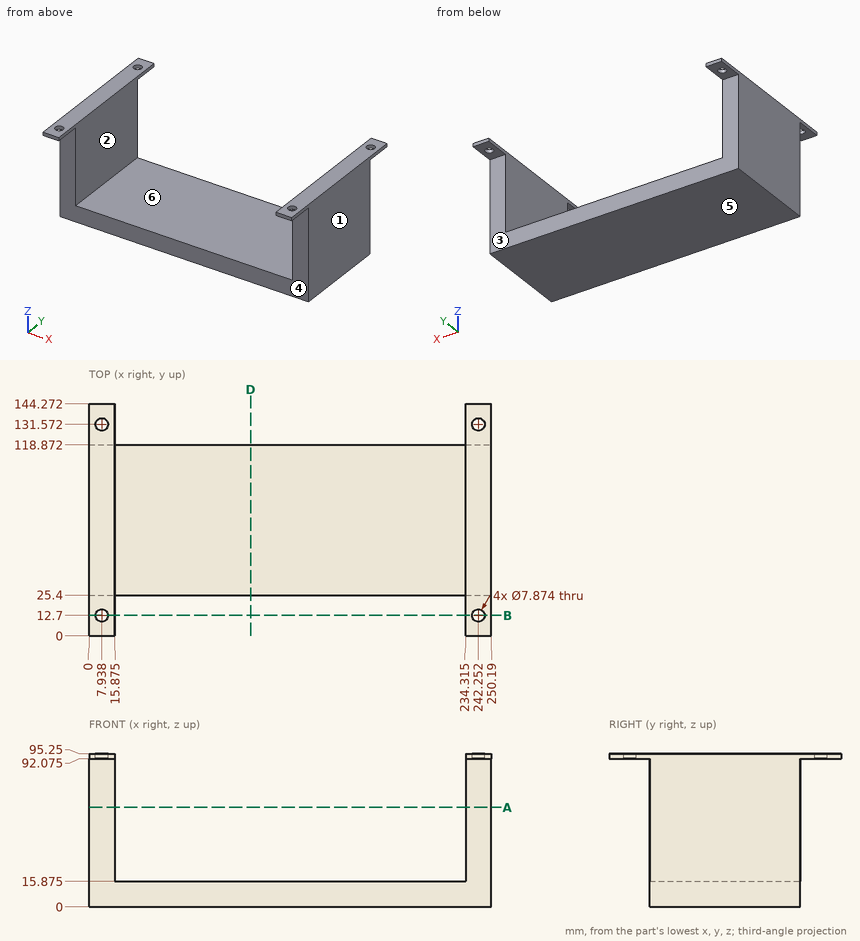
Input: dimensioned drawing with shaded views. Units: mm. Origin: part minimum x, y, z. A direction names the side the tool comes from. Give positions to 0.01 mm unless a question says otherwise; leave off trailing zeros. Loops run counter-clockwise (first coordinate to the right, second up) from the corner with the lowest first, then second, coordinate; pieces in that order, holes last. Notation, with made-up numbers: (-32.5, -17.75) -> (-21.5, -17.75) arc R21 cw to (-21.5, 16.25) -> close; hole circle Ø4 at (-13.5, -15.5). An arc over 180 degrees is marked (long way). Use a Markdown table: item, result.
Q1. Section query B-B, the plane y = 12.7. State how many separate pieces and enclosed holes the cut face has.
Entries:
| item | result |
|---|---|
| separate pieces | 4 |
| enclosed holes | 0 |
Q2. Ray query, probe 1 along X at (y, z) = (89, 41.5) (1 decimal); probe 2 along Z at (x, y) = (234, 40.5) (1 decimal); probe 3 along Y at (x, z) = (217, 9). Return the intervals inside material, ascending. Write a range as from..to.
Entries:
| item | result |
|---|---|
| probe 1 | x = 0..15.9, 234.3..250.2 |
| probe 2 | z = 0..15.9 |
| probe 3 | y = 25.4..118.87 |
Q3. Access query for the marked faces 4, 5 and 6. Directions: +Z, -Z, +X, -X, +Y, -Y. A direction counts if a zero-diameter tool reaches every point of the face in a straight line with its end or side. Return the directions, or none.
Entries:
| item | result |
|---|---|
| face 4 | -Z, +X, -X, -Y |
| face 5 | -Z, +X, -X, +Y, -Y |
| face 6 | +Z, +Y, -Y |
Q4. Section query D-D, the plane x = 100.5. Return the cut outline in (y, z) (1 decimal), plus the area to 3 significant figures.
Entries:
| item | result |
|---|---|
| outline | (25.4, 0) -> (118.9, 0) -> (118.9, 15.9) -> (25.4, 15.9) -> close |
| area | 1,480 mm² |
Q5. Pull-direction query (X, two-part tool) for the marked faces 1, 2 and 3; classes: pulls with the +X half, pulls with the -X half, needs draft (parallel to the pull), parting line crosses it, or undercut.
Entries:
| item | result |
|---|---|
| face 1 | pulls with the +X half |
| face 2 | undercut |
| face 3 | needs draft |
Q6. First-contact query: P1, Ø4, axis at y = 30.5, z = 26, coming from the -X side; P2, Ø3, axis at x = 53.5, y = 83.5, coming from the +Z side (1 decimal); P3, Ø17.5, axis at x = 9, y = 129, coming from the -Z side (1 decimal); P4, Ø3, axis at x = 208, z = 11, coming from the +Y side. Flat tips, straight axial feed; report the tip coordinate or a pass-through.
Entries:
| item | result |
|---|---|
| P1 | stops at x = 0 |
| P2 | stops at z = 15.9 |
| P3 | stops at z = 92.1 |
| P4 | stops at y = 118.87 |
Q7. Section query A-A, the plane z = 62. Return the cut outline in (x, y) (1 decimal), plus the area to 3 significant figures.
Entries:
| item | result |
|---|---|
| outline | (0, 25.4) -> (15.9, 25.4) -> (15.9, 118.9) -> (0, 118.9) -> close; (234.3, 25.4) -> (250.2, 25.4) -> (250.2, 118.9) -> (234.3, 118.9) -> close |
| area | 2,970 mm² |
